For this review, take the finished solid that the model builds, in its own axes (mm). A direction names the side the tool comes from. Round coordinates to 2 decimals unless told otherwise and drop trailing zeros. Use one line per item in the form item = value. Start each with the question number.
Item 1: For faces 4 (the cylindrical face through (9.401, 4.151, -1.635)), 5 (the cylindrical face through (10.593, 2.301, 1.635)), 6 (the cylindrical face through (-11.815, 6.648, 1.049)), list the 3-axis set-ups (+Z, -Z, +X, -X, +Y, -Y) from which the entire face can be reached by the end or side of a thin tool; tool diameter is ignored.
Item 2: Add section B-B (y = 6.2). Count the separate pieces of the cut face and the enclosed holes in it, and give its area (3 significant figures).
Item 3: For line 1 (X direction, y = 3, z = -4.25); line 2 (X direction, y = 6.2, z = -2); line 3 (X direction, y = 6.2, z = -1.25), list the stretches that pass through material, from the lowest coordinate up. Write a range as [from, to].
Item 4: For P1, Ø2.5, axis at x = 9.5, y = 4.5, coming from the -Z side; P2, Ø1, axis at y = 4, z = 4, coming from the +X side; P3, Ø0.7, axis at x = -8.5, y = 6, coming from the +Z side, all flat-tipped, find the tip position at first contact; note any pin that passes through.
Item 5: Draft analysis for pull direction X (two halves, no side actions). For faces 1 (the flat face through (-9, 5, -0.35)), 2 (the cylindrical face through (-9.385, 8.71, 1.651)), 3 (the cylindrical face through (9.385, 4.151, 1.651)), state which applies: released by +X, released by -X, zero draft, split by the parting line, or undercut.
from build123d import *

# Parameters (mm, degrees)
SKETCH1_W              = 30
SKETCH1_H              = 30
BOSS_EXTRUDE1_DEPTH    = 2
BOSS_EXTRUDE2_DEPTH    = 8.4
FILLET1_R              = 1
CUT_EXTRUDE1_START     = -6.566028302
CUT_EXTRUDE1_OUTLINE_R = 1
CUT_EXTRUDE1_DEPTH     = 10.432056604
SKETCH6_W              = 4
SKETCH6_H              = 3.8
CUT_EXTRUDE2_DEPTH     = 0.6
CUT_EXTRUDE3_START     = 16.2
SKETCH6_2_W            = 4
SKETCH6_2_H            = 3.8
CUT_EXTRUDE3_DEPTH     = 0.6
FILLET2_R              = 1


# Read off the part's stored shape, not the designer's step: Cut-Extrude1, Mirror1
# Some blends are built 0.0001 mm under size
with BuildPart() as part:
    # Sketch1 → Boss-Extrude1 (new body)
    with BuildSketch(Plane(origin=(0, 0, 0), x_dir=(1, 0, 0), z_dir=(0, 1, 0))):
        Rectangle(SKETCH1_W, SKETCH1_H)
    extrude(amount=BOSS_EXTRUDE1_DEPTH)

    # Sketch2 → Boss-Extrude2 (add)
    with BuildSketch(Plane(origin=(0, 2, 0), x_dir=(1, 0, 0), z_dir=(0, 1, 0))):
        Polygon((-9.1, 5.35), (-8.1, 5.35), (-8.1, 0.35), (-11.1, 0.35), (-11.1, -0.35), (-8.1, -0.35), (-8.1, -5.35), (-9.1, -5.35), (-9.1, -1.35), (-12.1, -1.35), (-12.1, 1.35), (-9.1, 1.35), align=None)
    extrude(amount=BOSS_EXTRUDE2_DEPTH)

    # Fillet1
    # the kernel refuses this fillet: 1 mm, written as the material it adds along each edge
    with BuildSketch(Plane(origin=(-9.1, 2, -1.35), x_dir=(0, 0, -1), z_dir=(0, 1, 0)), Plane(origin=(-9.1, 2, 1.35), x_dir=(-1, 0, 0), z_dir=(0, 1, 0))) as fillet1_piece_1:
        with BuildLine():
            CenterArc((FILLET1_R, FILLET1_R), FILLET1_R, 180, 90)
            Line((0, FILLET1_R), (0, 0))
            Line((0, 0), (FILLET1_R, 0))
        make_face()
    extrude(amount=8.4)
    # the kernel refuses this fillet: 1 mm, written as the material it takes off along each edge
    with BuildSketch(Plane(origin=(-9.1, 2, -5.35), x_dir=(1, 0, 0), z_dir=(0, 1, 0)), Plane(origin=(-12.1, 2, -1.35), x_dir=(1, 0, 0), z_dir=(0, 1, 0)), Plane(origin=(-12.1, 2, 1.35), x_dir=(0, 0, -1), z_dir=(0, 1, 0)), Plane(origin=(-9.1, 2, 5.35), x_dir=(0, 0, -1), z_dir=(0, 1, 0))) as fillet1_2_piece_1:
        with BuildLine():
            CenterArc((FILLET1_R, -FILLET1_R), FILLET1_R, 90, 90)
            Line((0, -FILLET1_R), (0, 0))
            Line((0, 0), (FILLET1_R, 0))
        make_face()
    extrude(amount=10.9, mode=Mode.SUBTRACT)
    # the kernel refuses this fillet: 1 mm, written as the material it adds along each edge
    with BuildSketch(Plane(origin=(-9.1, 2, -2.35), x_dir=(-1, 0, 0), z_dir=(0, 0, -1)), Plane(origin=(-9.1, 2, 4.35), x_dir=(-1, 0, 0), z_dir=(0, 0, -1))) as fillet1_3_piece_1:
        with BuildLine():
            CenterArc((FILLET1_R, FILLET1_R), FILLET1_R, 180, 90)
            Line((0, FILLET1_R), (0, 0))
            Line((0, 0), (FILLET1_R, 0))
        make_face()
    extrude(amount=2)
    with BuildSketch(Plane(origin=(-11.1, 2, -1.35), x_dir=(0, 0, -1), z_dir=(1, 0, 0)), Plane(origin=(-10.1, 2, 1.35), x_dir=(0, 0, 1), z_dir=(-1, 0, 0))) as fillet1_3_piece_2:
        with BuildLine():
            CenterArc((FILLET1_R, FILLET1_R), FILLET1_R, 180, 90)
            Line((0, FILLET1_R), (0, 0))
            Line((0, 0), (FILLET1_R, 0))
        make_face()
    extrude(amount=1)
    with BuildSketch(Plane(origin=(-12.1, 2, 0.35), x_dir=(-1, 0, 0), z_dir=(0, 0, -1))) as fillet1_3_piece_3:
        with BuildLine():
            CenterArc((FILLET1_R, FILLET1_R), FILLET1_R, 180, 90)
            Line((0, FILLET1_R), (0, 0))
            Line((0, 0), (FILLET1_R, 0))
        make_face()
    extrude(amount=0.7)
    with BuildSketch(Plane(origin=(-8.1, 2, 4.35), x_dir=(-1, 0, 0), z_dir=(0, 0, -1))) as fillet1_3_piece_4:
        with BuildLine():
            CenterArc((1 + FILLET1_R, FILLET1_R), FILLET1_R, 180, 90)
            Line((1, FILLET1_R), (1, 0))
            Line((1, 0), (1 + FILLET1_R, 0))
        make_face()
    revolve(axis=Axis((-8.1, 2, 4.35), (0, 1, 0)), revolution_arc=90)
    with BuildSketch(Plane(origin=(-10.1, 2, 2.35), x_dir=(0, 0, -1), z_dir=(-1, 0, 0))) as fillet1_3_piece_5:
        with BuildLine():
            CenterArc((1 - FILLET1_R, -FILLET1_R), FILLET1_R, 0, 90)
            Line((1, -FILLET1_R), (1, 0))
            Line((1, 0), (1 - FILLET1_R, 0))
        make_face()
    revolve(axis=Axis((-10.1, 2, 2.35), (0, -1, 0)), revolution_arc=90)
    with BuildSketch(Plane(origin=(-11.1, 2, 0.35), x_dir=(-1, 0, 0), z_dir=(0, 0, -1))) as fillet1_3_piece_6:
        with BuildLine():
            CenterArc((1 + FILLET1_R, FILLET1_R), FILLET1_R, 180, 90)
            Line((1, FILLET1_R), (1, 0))
            Line((1, 0), (1 + FILLET1_R, 0))
        make_face()
    revolve(axis=Axis((-11.1, 2, 0.35), (0, 1, 0)), revolution_arc=90)
    with BuildSketch(Plane(origin=(-11.1, 2, -0.35), x_dir=(0, 0, -1), z_dir=(1, 0, 0))) as fillet1_3_piece_7:
        with BuildLine():
            CenterArc((1 + FILLET1_R, FILLET1_R), FILLET1_R, 180, 90)
            Line((1, FILLET1_R), (1, 0))
            Line((1, 0), (1 + FILLET1_R, 0))
        make_face()
    revolve(axis=Axis((-11.1, 2, -0.35), (0, 1, 0)), revolution_arc=90)
    with BuildSketch(Plane(origin=(-10.1, 2, -2.35), x_dir=(1, 0, 0), z_dir=(0, 0, -1))) as fillet1_3_piece_8:
        with BuildLine():
            CenterArc((1 - FILLET1_R, -FILLET1_R), FILLET1_R, 0, 90)
            Line((1, -FILLET1_R), (1, 0))
            Line((1, 0), (1 - FILLET1_R, 0))
        make_face()
    revolve(axis=Axis((-10.1, 2, -2.35), (0, -1, 0)), revolution_arc=90)
    with BuildSketch(Plane(origin=(-8.1, 2, -4.35), x_dir=(0, 0, -1), z_dir=(1, 0, 0))) as fillet1_3_piece_9:
        with BuildLine():
            CenterArc((1 + FILLET1_R, FILLET1_R), FILLET1_R, 180, 90)
            Line((1, FILLET1_R), (1, 0))
            Line((1, 0), (1 + FILLET1_R, 0))
        make_face()
    revolve(axis=Axis((-8.1, 2, -4.35), (0, 1, 0)), revolution_arc=90)

    # Cut-Extrude1 outline → Cut-Extrude1 (cut)
    with BuildSketch(Plane.XY.offset(1.35).offset(CUT_EXTRUDE1_START)):
        with Locations((-9.6, 6.2)):
            Circle(CUT_EXTRUDE1_OUTLINE_R)
    extrude(amount=CUT_EXTRUDE1_DEPTH, mode=Mode.SUBTRACT)

    # Mirror1: part across plane


with BuildPart() as part_1:
    add(part.part)
    add(part.part.mirror(Plane(origin=(0, 0, 0), x_dir=(0, 0, 1), z_dir=(1, 0, 0))))

    # Sketch6 → Cut-Extrude2 (cut)
    with BuildSketch(Plane.ZY.offset(-8.1)):
        with Locations((3.35, 6.2)):
            Rectangle(SKETCH6_W, SKETCH6_H)
    extrude(amount=-CUT_EXTRUDE2_DEPTH, mode=Mode.SUBTRACT)

    # Sketch6<2> → Cut-Extrude3 (cut)
    with BuildSketch(Plane.ZY.offset(-8.1).offset(CUT_EXTRUDE3_START)):
        with Locations((3.35, 6.2)):
            Rectangle(SKETCH6_2_W, SKETCH6_2_H)
    extrude(amount=CUT_EXTRUDE3_DEPTH, mode=Mode.SUBTRACT)

    # Fillet2
    fillet2_edges = [part_1.edges().sort_by_distance(p)[0] for p in [
        (-15, 2, 0),
        (0, 2, 15),
        (15, 2, 0),
        (0, 0, 15),
        (-15, 0, 0),
        (0, 0, -15),
        (15, 0, 0),
        (15, 1, 15),
        (-15, 1, 15),
        (-15, 1, -15),
        (15, 1, -15),
        (0, 2, -15),
    ]]
    fillet(fillet2_edges, radius=FILLET2_R - 0.0001)  # a hair under: the kernel refuses the full size


solid = part_1.part
Calculated:
q1.face_4 = -Z, +X, +Y
q1.face_5 = +Z, +X, +Y
q1.face_6 = +Z, -X, +Y
q2.separate_pieces = 6
q2.enclosed_holes = 0
q2.area = 12.5 mm^2
q3.line_1 = [-9.1, -8.1], [8.1, 9.1]
q3.line_2 = [-8.6, -8.1], [8.1, 8.6]
q3.line_3 = [-11.54, -10.6], [-8.6, -8.1], [8.1, 8.6], [10.6, 11.54]
q4.P1 = -5.34
q4.P2 = 9.1
q4.P3 = 5.15
q5.face_1 = undercut
q5.face_2 = released by -X
q5.face_3 = released by +X
